Autodesk Inventor part; units mm, degrees
ref_plane "Work Plane1" through (0, 0, 0) normal (0, -1, 0) x (1, 0, 0)
ref_plane "YZ Plane" through (0, 0, 0) normal (1, 0, 0) x (0, 1, 0)
ref_plane "XZ Plane" through (0, 0, 0) normal (0, 1, 0) x (-1, 0, 0)
sketch "Sketch1" plane through (0, 0, 0) normal (1, 0, 0) x (0, 1, 0)
  circle A0 centre (0, 0) radius 5.9
  circle A1 centre (0, 0) radius 3.25
  dimension "d0" = 6.5
  dimension "d1" = 11.8
extrude "Body" add sketch "Sketch1" along normal blind 1.3
fillet "Fillet" radius 0.3 2 edges at (1.3, -3.25, 0) (0, -3.25, 0)
sketch "Sketch2" plane through (0, 0, 0) normal (0, 0, 1) x (1, 0, 0)
  line L0 (0, -3.25) -> (0, 3.25)
  line L1 (1.3, 5.9) -> (1.3, -5.9)
  line L2 (-1.2, 0) -> (7.2, 0)
  line L3 (0, -0.26) -> (1.3, 0.4906)
  line L4 (0, 0.26) -> (1.3, 1.0106)
  dimension "d4" = 0.26
  dimension "d5" = 0.26
  dimension "d6" = 60
extrude "Cut" cut sketch "Sketch2" along normal up to next contours L0 L2 L3 | L0 L4 L1 L3 L2
ref_plane "Work Plane1" through (0, 0, 0) normal (0, -1, 0) x (1, 0, 0)
equation "\"d0\" = SD1"
equation "\"d1\" = SD2"
equation "\"d2\" = SD"
equation "\"d4\" = 0.2 * SD"
equation "\"d5\" = 0.2 * SD"
equation "\"d6\" = FAWI"
equation "\"d7\" = SD"
equation "\"d13\" = R"
equation "\"SD1\" = 6.5"
equation "\"SD2\" = 11.8"
equation "\"SD\" = 1.3"
equation "\"FAWI\" = 60deg"
equation "\"R\" = 0.3"
equation "\"NND\" = 6"
properties part number "DIN 128 - A6" material "Steel, Mild"
The model under review builds one solid part; all positions refer to its coordinate system, in mm. Give positions to 0.01 mm unless a question says otherwise; leave off trailing zeros. Order: outer loops, then holes, each group sorted by start corner. A loop starts at its lowest first (then second) coordinate and runs counter-clockwise, first axis right, second up. Notation, with made-up numbers: M -14,14 L 30,14 A7 cw 30,18 Z; hole C 45,40 d5. An arc over 180 degrees is marked long. One line per question, with ' | ' between items. Start each with the question number.
1) Consider section C-C, the plane x = 0.5. Give the boundary of the cut face in (y, z).
2) Consider section B-B, the plane y = -4.75. Give the boundary of the cut face in (x, z), then the cut area to 3 significant figures.
3) Consider section A-A, the plane z = 4. Give the boundary of the cut face in (x, y).
4) Mouldability with a two-part tool opening along X and no side actions: class faces 1 (the face through (0.64, 0.11, 4.55)), 2 (the face through (1.3, 3, -3)), 3 (the face through (0, 3, -3)), 4 (the face through (0.64, 0.63, 4.49)) as pulls with the +X half, pulls with the -X half, needs draft (parallel to the pull), parting line crosses it, or undercut.
5) Wall thickness on L1, parallel to Z at x = 0.7, y = 0; L2, parallel to Y at x = 1.05, z = 2: over which ranges is each line inside the solid? List them lowest first. Write a range as from..to.
Found:
1) outline: M 0.03,3.25 L 0.03,5.9 A5.9 ccw long 0.55,5.87 L 0.55,3.2 A3.25 cw long Z
2) outline: M 0,-3.5 L 1.3,-3.5 L 1.3,3.5 L 0,3.5 Z | area: 9.10 mm²
3) outline: M 0,-4.34 L 1.3,-4.34 L 1.3,0.49 L 0,-0.26 Z; M 0,0.26 L 1.3,1.01 L 1.3,4.34 L 0,4.34 Z
4) face 1: undercut | face 2: pulls with the +X half | face 3: pulls with the -X half | face 4: undercut
5) L1: z = -5.9..-3.25, 3.25..5.9 | L2: y = -5.55..-2.57, 2.57..5.55
